Input: part model. Units: mm. Frame: model coordinates. Face numbers are marked on the shaded views. A direction names the side the tool comes from. Coordinates: 2 decimals unless noted, no trailing zeros. Order: outer loops, then holes, each group sorted by start corner. A loop starts at its lowest first (then second) coordinate and runs counter-clockwise, first axis right, second up.
from build123d import *

# Parameters (mm, degrees)
SKETCH1_R            = 7
SKETCH1_R_2          = 5
BOSS_EXTRUDE1_DEPTH  = 3.25
SKETCH2_R            = 9
SKETCH2_R_2          = 5
BOSS_EXTRUDE2_DEPTH  = 2.5
FILLET1_R            = 2
FILLET1_OF_MIRROR1_R = 2


with BuildPart() as part:
    # Sketch1 → Boss-Extrude1 (new, symmetric)
    with BuildSketch(Plane.XY):
        with Locations(Location((0, 0, 0), (0, 0, 180))):
            Circle(SKETCH1_R)
        with Locations(Location((0, 0, 0), (0, 0, 180))):
            Circle(SKETCH1_R_2, mode=Mode.SUBTRACT)
    extrude(amount=BOSS_EXTRUDE1_DEPTH, both=True)

    # Sketch2 → Boss-Extrude2 (add)
    with BuildSketch(Plane.XY.offset(3.25)):
        Circle(SKETCH2_R)
        with Locations(Location((0, 0, 0), (0, 0, 180))):
            Circle(SKETCH2_R_2, mode=Mode.SUBTRACT)
    boss_extrude2 = extrude(amount=BOSS_EXTRUDE2_DEPTH)

    # Fillet1
    fillet1_edges = [part.edges().sort_by_distance(p)[0] for p in [
        (-9, 0, 5.75),
    ]]
    fillet(fillet1_edges, radius=FILLET1_R)

    # Mirror1: Boss-Extrude2 across plane
    add(boss_extrude2.mirror(Plane.XY))

    # Fillet1 of Mirror1
    fillet1_of_mirror1_edges = [part.edges().sort_by_distance(p)[0] for p in [
        (-9, 0, -5.75),
    ]]
    fillet(fillet1_of_mirror1_edges, radius=FILLET1_OF_MIRROR1_R)


solid = part.part
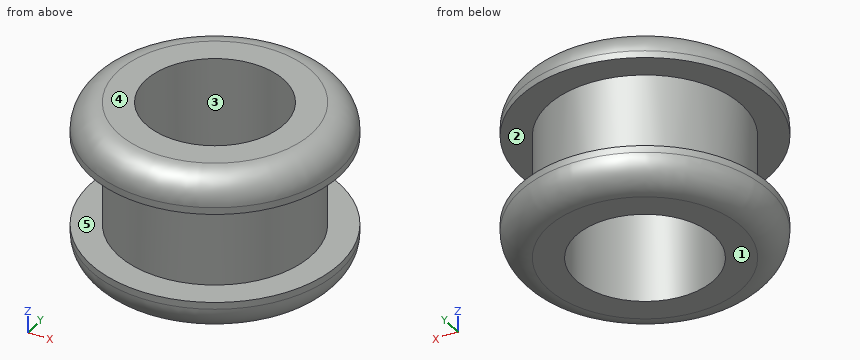
Item 1: Cut plane D-D on z = -4.25. Return loops of the section in (x, y).
Response values:
outline: circle Ø17.87 at (0, 0); hole circle Ø10 at (0, 0)
Item 2: Pin query (flat end, axial travel): pin 1 Ø1 at (x, z) = (-5, -4.5) entering from -Y; pin 2 Ø1 at (x, z) = (5.5, 3) entering from +Y; pin 3 Ø1 at (y, z) = (6.5, 3) entering from +X. Return the tip coordinate at first contact, or that it passes through.
Response values:
pin 1: stops at y = -7.68
pin 2: stops at y = 7.44
pin 3: stops at x = 6.65
Item 3: Draft query along Z for the marked faces 3, 4 and 5. Return one class per face: pulls with the +Z half, pulls with the -Z half, needs draft (parallel to the pull), parting line crosses it, or undercut.
Response values:
face 3: needs draft
face 4: pulls with the +Z half
face 5: undercut
Item 4: Cut plane C-C on z = 2.75. Return loops of the section in (x, y), then the cut area to 3 significant figures.
Response values:
outline: circle Ø14 at (0, 0); hole circle Ø10 at (0, 0)
area: 75.4 mm2
Item 5: Cut plane A-A on x = 0. Return loops of the section in (y, z).
Response values:
outline: (-9, -3.75) arc R2 ccw to (-7, -5.75) - (-5, -5.75) - (-5, 5.75) - (-7, 5.75) arc R2 ccw to (-9, 3.75) - (-9, 3.25) - (-7, 3.25) - (-7, -3.25) - (-9, -3.25) - close; (5, -5.75) - (7, -5.75) arc R2 ccw to (9, -3.75) - (9, -3.25) - (7, -3.25) - (7, 3.25) - (9, 3.25) - (9, 3.75) arc R2 ccw to (7, 5.75) - (5, 5.75) - close
Item 6: Ray query, probe 1 along Y at (x, z) = (0, -0.5); probe 2 along X at (y, z) = (-4.25, -1.5); probe 3 along Z at (x, y) = (7.5, 1). Return the intervals inside material, ascending.
Response values:
probe 1: y = -7 to -5, 5 to 7
probe 2: x = -5.56 to -2.63, 2.63 to 5.56
probe 3: z = -5.67 to -3.25, 3.25 to 5.67
Item 7: Access query for the marked faces 1 and 2. Directions: +Z, -Z, +X, -X, +Y, -Y. A direction counts if a zero-diameter tool reaches every point of the face in a straight line with its end or side. Return the directions, or none.
Response values:
face 1: -Z, +X, -X, +Y, -Y
face 2: none
